```python
from build123d import *

# Parameters (mm, degrees)
F0_W      = 70
F0_H      = 330
F1_DEPTH  = 120
F2_W      = 60
F2_H      = 280
F3_DEPTH  = 60
F4_R      = 27.5
F5_DEPTH  = 30
F6_W      = 60
F6_H      = 55
F7_DEPTH  = 25
F8_W      = 10
F8_H      = 25
F9_DEPTH  = 25
F10_DEPTH = 25
F11_SIZE  = 5
F12_SIZE  = 5


with BuildPart() as f1:
    # F0 (on Top) → F1 (new body)
    with BuildSketch(Plane.XY):
        with Locations((-0.983767, 35.842364)):
            Rectangle(F0_W, F0_H)
    extrude(amount=F1_DEPTH)

    # F2 (on face) → F3 (cut)
    with BuildSketch(Plane.XY.offset(120)):
        with Locations((-5.983767, 35.842364)):
            Rectangle(F2_W, F2_H)
    extrude(amount=-F3_DEPTH, mode=Mode.SUBTRACT)

    # F4 (on face) → F5 (cut)
    with BuildSketch(Plane.XY.offset(60)):
        with Locations((-9.620236, -74.157636)):
            Circle(F4_R)
    extrude(amount=-F5_DEPTH, mode=Mode.SUBTRACT)

    # F6 (on face) → F7 (cut, through all)
    with BuildSketch(Plane.XZ.offset(129.157636)):
        with Locations((-5.983767, 92.5)):
            Rectangle(F6_W, F6_H)
    extrude(amount=-F7_DEPTH, mode=Mode.SUBTRACT)

    # F8 (on face) → F9 (join)
    with BuildSketch(Plane.XY.offset(65)):
        with Locations((-30.983767, -116.657636)):
            Rectangle(F8_W, F8_H)
    extrude(amount=F9_DEPTH)

    # F8 (on face) → F10 (join)
    with BuildSketch(Plane.XY.offset(65)):
        with Locations((19.016233, -116.657636)):
            Rectangle(F8_W, F8_H)
    extrude(amount=F10_DEPTH)

    # F11
    f11_edges = [f1.edges().sort_by_distance(p)[0] for p in [
        (14.016233, -116.657636, 90),
    ]]
    chamfer(f11_edges, length=F11_SIZE)

    # F12
    f12_edges = [f1.edges().sort_by_distance(p)[0] for p in [
        (-25.983767, -116.657636, 90),
    ]]
    chamfer(f12_edges, length=F12_SIZE)


solid = f1.part
```
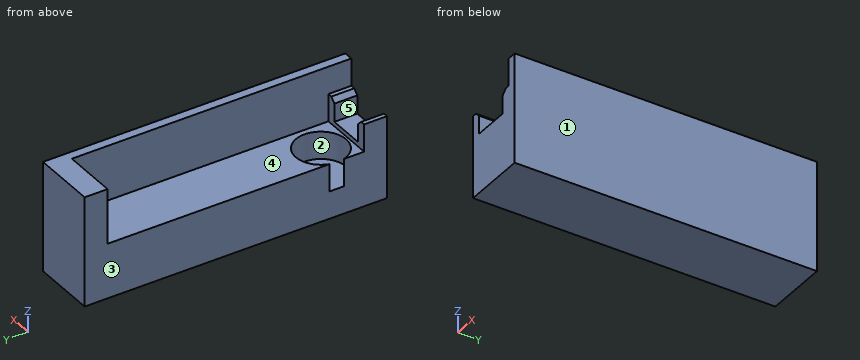
For this review, take the finished solid that the model builds, in its own axes (mm). Face numbers are marked on the shaded views. A direction names the side the tool comes from. Round coordinates to 2 decimals unless told otherwise and drop trailing zeros. Write each loop counter-clockwise with the first axis right and the second up, starting at its lowest first coordinate (ties: lowest second). Pieces come first, ordered by that corner, then holes. Notation, with made-up numbers: (47, -28.5) - (77, -28.5) arc R20 ccw to (77, 4.5) - close; hole circle Ø2 at (85, -16). An arc over 180 degrees is marked (long way). Answer as CSV lines item,"result". Start each with the question number.
(1) Machinability: for the marked faces 1 and 2, which of the approach directions +Z, -Z, +X, -X, +Y, -Y give a long, thin tool a straight path to every point of the face, cutting with its end or side? Answer none if there is none.
(2) For pin 1 (2 mm diameter, centred on y = 119, z = 69, fed in from -X); pin 2 (1.5 mm diameter, centred on x = 21, y = -112.5, fed in from +Z); pin 3 (16 mm diameter, centred on x = -6, y = -82, fed in from +Z); pin 4 (4 mm diameter, centred on x = -14, y = -10, fed in from -Z), all flat-tipped, find the tip position at first contact; note any pin that passes through.
(3) Add section B-B, the plane z = 101.5. State the section outline as (x, y) points, plus the area to 3 significant figures.
(4) Add section C-C, the plane y = 120. State the section outline as (x, z) points, plus the area to 3 significant figures.
(5) Add section D-D, the plane x = -0.5. State the section outline as (y, z) points.
(6) Mouldability with a two-part tool opening along X and no side actions: class the marked faces 3, 4 and 5 as +X half, -X half, draft (parallel to the pull), parting line (faces both ways), or undercut.
(7) Add section A-A, the plane x = -18. State the section outline as (y, z) points, plus the area to 3 significant figures.
(8) For line 1 (Y direction, x = -26.5, z = 67); line 2 (Y direction, x = 0, z = 107); line 3 (Z direction, x = 12, y = 8.5), list the stretches that pass through material, from the lowest coordinate up.
From the geometry:
1,face 1,"+Z, -Z, +X, +Y, -Y"
1,face 2,"+Z"
2,pin 1,"stops at x = 24.02"
2,pin 2,"stops at z = 90"
2,pin 3,"stops at z = 30"
2,pin 4,"stops at z = 0"
3,outline,"(-35.98, 175.84) - (24.02, 175.84) - (24.02, -129.16) - (34.02, -129.16) - (34.02, 200.84) - (-35.98, 200.84) - close"
3,area,"4,800 mm²"
4,outline,"(-35.98, 0) - (34.02, 0) - (34.02, 120) - (24.02, 120) - (24.02, 60) - (-35.98, 60) - close"
4,area,"4,800 mm²"
5,outline,"(-129.16, 0) - (200.84, 0) - (200.84, 120) - (175.84, 120) - (175.84, 60) - (-48.21, 60) - (-48.21, 30) - (-100.1, 30) - (-100.1, 60) - (-104.16, 60) - (-104.16, 65) - (-129.16, 65) - close"
6,face 3,"-X half"
6,face 4,"draft"
6,face 5,"undercut"
7,outline,"(-129.16, 0) - (200.84, 0) - (200.84, 120) - (175.84, 120) - (175.84, 60) - (-47.97, 60) - (-47.97, 30) - (-100.35, 30) - (-100.35, 60) - (-104.16, 60) - (-104.16, 65) - (-129.16, 65) - close"
7,area,"19,900 mm²"
8,line 1,"y = -129.16 to -104.16, 175.84 to 200.84"
8,line 2,"y = 175.84 to 200.84"
8,line 3,"z = 0 to 60"
